Model file for the job. Use its own axes, mm. Face numbers are marked on the shaded views. A direction names the side the tool comes from. Coordinates: 2 decimals unless noted, no trailing zeros. Write each loop counter-clockwise with the first axis right and the second up, starting at its lowest first coordinate (ties: lowest second). Pieces come first, ordered by that corner, then holes. Notation, with made-up numbers: M -39,83 L 4,83 A12 ccw 4,105 Z; hole C 16.5,38 d4. An arc over 180 degrees is marked long. One line per question, with ' | ' between items. Start each with the question number.
(1) Tool access for the marked faces 1, 2 and 3: list every direction of +Z, -Z, +X, -X, +Y, -Y with a clear straight run to the whole face (end or side of a thin tool).
(2) Cut at C-C (x = 12.5). Write the cut outline in (y, z), plus the area to 3 significant figures.
(3) Cut at D-D (z = -12). Write the cut outline in (x, y), plus the area to 3 significant figures.
(4) Flat gauge pins, fed straight in: pin 1 Ø5.5 at (x, z) = (12.5, 0) entering from +Y; pin 2 Ø3 at (x, z) = (-1, 0.5) entering from -Y; pin 3 Ø5 at (x, y) = (-4, 20.5) entering from +Z; pin 4 Ø1.5 at (x, z) = (5, -12.5) entering from -Y. Where does each tip first touch, or does it go through?
(5) Cut at A-A (x = 0). Write the cut outline in (y, z).
(6) Wall check: probe 1 along Z at (x, y) = (0, 2); probe 2 along X at (y, z) = (3, -12); probe 3 along Z at (x, y) = (-12.5, 4.75). Give the ranges that are in metal, low to high.
(7) Two-plate mould, pull along X, no slides. Class the marked faces 4, 5 and 6: +X half, -X half, draft (parallel to the pull), parting line (faces both ways), or undercut.
(8) Cut at B-B (z = 0). Write the cut outline in (x, y), plus the area to 3 significant figures.
from build123d import *

# Parameters (mm, degrees)
SKETCH1_R           = 16.5
BOSS_EXTRUDE1_DEPTH = 7
SKETCH2_R           = 1.75
CUT_EXTRUDE1_DEPTH  = 8
CIRPATTERN1_COUNT   = 4
SKETCH3_R           = 5
BOSS_EXTRUDE2_DEPTH = 25
CHAMFER1_SIZE       = 4
SKETCH6_R           = 5.25
CUT_EXTRUDE4_DEPTH  = 5.5
SKETCH8_R           = 2.75
CUT_EXTRUDE5_DEPTH  = 6


with BuildPart() as part:
    # Sketch1 → Boss-Extrude1 (new body)
    with BuildSketch(Plane(origin=(0, 0, 0), x_dir=(1, 0, 0), z_dir=(0, 1, 0))):
        Circle(SKETCH1_R)
    extrude(amount=BOSS_EXTRUDE1_DEPTH)

    # Sketch2 → Cut-Extrude1 (cut, through all)
    with BuildSketch(Plane(origin=(0, 7, 0), x_dir=(1, 0, 0), z_dir=(0, 1, 0))):
        with Locations((0, 12.5)):
            Circle(SKETCH2_R)
    cut_extrude1 = extrude(amount=-CUT_EXTRUDE1_DEPTH, mode=Mode.SUBTRACT)

    # CirPattern1: Cut-Extrude1 ×4 about axis
    cirpattern1_axis = Axis((0, 0, 0), (0, 1, 0))
    for i in range(1, CIRPATTERN1_COUNT):
        add(cut_extrude1.rotate(cirpattern1_axis, i * 360 / CIRPATTERN1_COUNT), mode=Mode.SUBTRACT)

    # Sketch3 → Boss-Extrude2 (add)
    with BuildSketch(Plane(origin=(0, 7, 0), x_dir=(1, 0, 0), z_dir=(0, 1, 0))):
        Circle(SKETCH3_R)
    extrude(amount=BOSS_EXTRUDE2_DEPTH)

    # Chamfer1
    chamfer1_edges = [part.edges().sort_by_distance(p)[0] for p in [
        (-5, 7, 0),
    ]]
    chamfer(chamfer1_edges, length=CHAMFER1_SIZE)

    # Sketch6 → Cut-Extrude4 (cut)
    with BuildSketch(Plane.XZ):
        Circle(SKETCH6_R)
    extrude(amount=-CUT_EXTRUDE4_DEPTH, mode=Mode.SUBTRACT)

    # Sketch8 → Cut-Extrude5 (cut)
    with BuildSketch(Plane.XZ.offset(-5.5)):
        Circle(SKETCH8_R)
    extrude(amount=-CUT_EXTRUDE5_DEPTH, mode=Mode.SUBTRACT)


solid = part.part
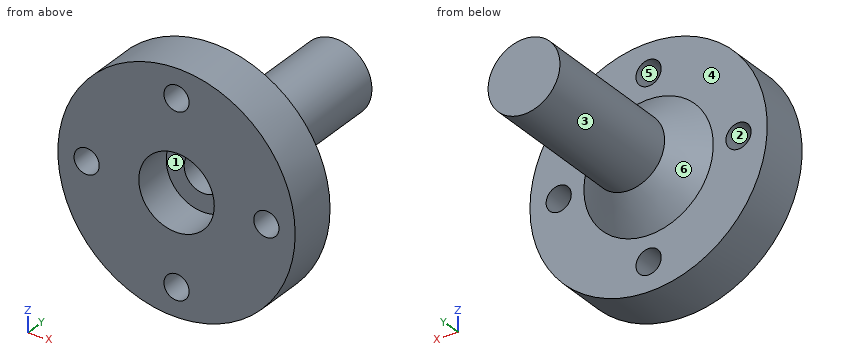
Filled in:
1) face 1: -Y | face 2: +Y, -Y | face 3: +Y
2) outline: M 0,-10.77 L 7,-10.77 L 7,-1.75 L 0,-1.75 Z; M 0,1.75 L 7,1.75 L 7,10.77 L 0,10.77 Z | area: 126 mm²
3) outline: M -11.32,0 L -1.68,0 L -1.68,7 L -11.32,7 Z; M 1.68,0 L 11.32,0 L 11.32,7 L 1.68,7 Z | area: 135 mm²
4) pin 1: y = 7 | pin 2: y = 11.5 | pin 3: z = 4.77 | pin 4: y = 0
5) outline: M 0,-16.5 L 7,-16.5 L 7,-14.25 L 0,-14.25 Z; M 0,-10.75 L 7,-10.75 L 7,-9 L 11,-5 L 32,-5 L 32,5 L 11,5 L 7,9 L 7,10.75 L 0,10.75 L 0,5.25 L 5.5,5.25 L 5.5,2.75 L 11.5,2.75 L 11.5,-2.75 L 5.5,-2.75 L 5.5,-5.25 L 0,-5.25 Z; M 0,14.25 L 7,14.25 L 7,16.5 L 0,16.5 Z
6) probe 1: -16.5 to -14.25, -10.75 to -5.25, 5.25 to 10.75, 14.25 to 16.5 | probe 2: -11.32 to -1.68, 1.68 to 11.32 | probe 3: -10.77 to -1.75, 1.75 to 10.77
7) face 4: draft | face 5: undercut | face 6: parting line
8) outline: M -16.5,0 L -14.25,0 L -14.25,7 L -16.5,7 Z; M -10.75,0 L -5.25,0 L -5.25,5.5 L -2.75,5.5 L -2.75,11.5 L 2.75,11.5 L 2.75,5.5 L 5.25,5.5 L 5.25,0 L 10.75,0 L 10.75,7 L 9,7 L 5,11 L 5,32 L -5,32 L -5,11 L -9,7 L -10.75,7 Z; M 14.25,0 L 16.5,0 L 16.5,7 L 14.25,7 Z | area: 357 mm²
